from build123d import *

# Parameters (mm, degrees)
F0_R           = 25
F1_DEPTH       = 25.4
F1_TAPER       = -30
F3_R           = 39.5485289591
F4_DEPTH       = 10.16
F6_R           = 20.0377303014
F7_DEPTH       = 35.5610001
F7_TAPER       = -1.5
F8_R           = 1.8145667082
F9_DEPTH       = 12.7
F9_DEPTH_BACK  = 25.4
F8_R_2         = 1.8161
F10_DEPTH      = 12.7
F10_DEPTH_BACK = 12.7
F11_DEPTH      = 12.7


# Not quite as in the source:
# - a fillet or chamfer that OpenCascade refuses, or shapes differently, is made with other operations: its cross-section is extruded or revolved along the edge and cut away or added


with BuildPart() as f1:
    # F0 (on Front) → F1 (new body)
    with BuildSketch(Plane.XZ):
        Circle(F0_R)
    extrude(amount=F1_DEPTH, taper=F1_TAPER)

    # F3 (on offset) → F4 (join)
    with BuildSketch(Plane.XZ.offset(25.4)):
        Circle(F3_R)
    extrude(amount=F4_DEPTH)

    # F5: fillet of radius 39.497 on 1 edges, made by hand

    # F5_s1 → F5_t2 (revolve, cut)
    with BuildSketch(Plane.XY):
        with BuildLine():
            ThreePointArc((39.5485289591, -25.4), (27.2681504962, -32.9326114571), (13.1032375067, -35.56))
            Line((13.1032375067, -35.56), (13.1032375067, -36.34994))
            Line((13.1032375067, -36.34994), (39.5485289591, -36.34994))
            Line((39.5485289591, -36.34994), (40.3384689591, -35.56))
            ThreePointArc((40.3384689591, -35.56), (40.3384689591, -30.48), (40.0774347881, -25.98674))
            Line((40.0774347881, -25.98674), (39.5485289591, -25.4))
        make_face()
    revolve(axis=Axis((0, -35.56, 0), (0, -1, 0)), mode=Mode.SUBTRACT)

    # F6 (on Front) → F7 (cut, through all)
    with BuildSketch(Plane.XZ):
        Circle(F6_R)
    extrude(amount=F7_DEPTH, taper=F7_TAPER, mode=Mode.SUBTRACT)

    # F8 (on Front) → F9 (cut, two sides)
    with BuildSketch(Plane.XZ) as f9_sk:
        with Locations((0, 22.6314)):
            Circle(F8_R)
    extrude(amount=F9_DEPTH, mode=Mode.SUBTRACT)
    extrude(f9_sk.sketch, amount=-F9_DEPTH_BACK, mode=Mode.SUBTRACT)

    # F8 (on Front) → F10 (cut, two sides)
    with BuildSketch(Plane.XZ) as f10_sk:
        with Locations((22.6314, 0)):
            Circle(F8_R_2)
    extrude(amount=-F10_DEPTH, mode=Mode.SUBTRACT)
    extrude(f10_sk.sketch, amount=F10_DEPTH_BACK, mode=Mode.SUBTRACT)

    # F8 (on Front) → F11 (cut)
    with BuildSketch(Plane.XZ):
        with Locations((0, 22.6314)):
            Circle(F8_R)
        with Locations((22.6314, 0)):
            Circle(F8_R_2)
        with Locations((0, -22.6314)):
            Circle(F8_R_2)
        with Locations((-22.6314, 0)):
            Circle(F8_R_2)
    extrude(amount=F11_DEPTH, mode=Mode.SUBTRACT)


solid = f1.part
Can you work these out from the model? Positions are in its coordinate system, mm. A direction names the side the tool comes from. Give positions to 0.01 mm unless a question says otherwise; leave off trailing zeros. One line per item, written item: value.
1) On a 3-axis mill with a long thin cutter (end or side, diameter ignored), from which of +Z, -Z, +X, -X, +Y, -Y can I reach the whole of each face in a straight line? I mean faces 4 (the face through (0.976, -6.261, -21.1)), 5 (the face through (-4.444, -17.63, -20.012)). Say none if no direction works.
Geometry check:
face 4: +Y
face 5: -Y
2) I'm going to push flat-ended pins straight in: pin 1 (6 mm diameter, centred on y = -22, z = 7, fed in from +X); pin 2 (4 mm diameter, centred on x = 21.5, y = -9.5, fed in from +Z); pin 3 (8 mm diameter, centred on x = -28, z = 4, fed in from -Y); pin 4 (8 mm diameter, centred on x = -11.5, z = -9, fed in from -Y). Where does each tip first touch, or does it pass through?
Geometry check:
pin 1: stops at x = 38.88
pin 2: stops at z = 24.01
pin 3: stops at y = -33.94
pin 4: passes through
3) Please list where these lines run through material, in increasing order: line 1 (Z direction, x = 0, y = -9.25); line 2 (X direction, y = -3.5, z = -4); line 3 (X direction, y = -3.5, z = -15).
Geometry check:
line 1: z = -30.34 to -24.45, -20.82 to -20.28, 20.28 to 20.82, 24.45 to 30.34
line 2: x = -26.72 to -19.73, 19.73 to 26.72
line 3: x = -22.47 to -13.42, 13.42 to 22.47
4) Thinking about a two-plate mould opening in Z: for faces 1 (the face through (-17, 0, -11)), 2 (the face through (-25.9, -1.6, 1.1)), 3 (the face through (0, -12.7, 23)), which applies, +Z half, -Z half, draft (parallel to the pull), parting line (faces both ways), or undercut?
Geometry check:
face 1: draft
face 2: parting line
face 3: undercut
